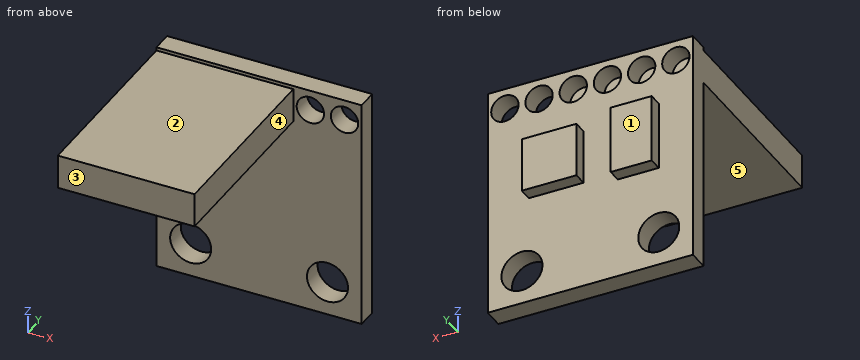
from build123d import *

# Parameters (mm, degrees)
ESQUISSE1_W        = 15
ESQUISSE1_H        = 17
ESQUISSE1_R        = 1.5
ESQUISSE1_R_2      = 1
BOSS_EXTRU_1_DEPTH = 1.5
ESQUISSE2_W        = 3
ESQUISSE2_H        = 5
ESQUISSE2_W_2      = 4
ESQUISSE2_H_2      = 4
BOSS_EXTRU_2_DEPTH = 1
ESQUISSE3_W        = 10
ESQUISSE3_H        = 2.5
BOSS_EXTRU_3_DEPTH = 14


with BuildPart() as part:
    # Esquisse1 → Boss.-Extru.1 (new body)
    with BuildSketch(Plane(origin=(0, 0, 0), x_dir=(1, 0, 0), z_dir=(0, 1, 0))):
        Rectangle(ESQUISSE1_W, ESQUISSE1_H)
        with Locations((-5, 6)):
            Circle(ESQUISSE1_R, mode=Mode.SUBTRACT)
        with Locations((5, 6)):
            Circle(ESQUISSE1_R, mode=Mode.SUBTRACT)
        with Locations((-6.25, -7)):
            Circle(ESQUISSE1_R_2, mode=Mode.SUBTRACT)
        with Locations((-3.75, -7)):
            Circle(ESQUISSE1_R_2, mode=Mode.SUBTRACT)
        with Locations((-1.25, -7)):
            Circle(ESQUISSE1_R_2, mode=Mode.SUBTRACT)
        with Locations((1.25, -7)):
            Circle(ESQUISSE1_R_2, mode=Mode.SUBTRACT)
        with Locations((3.75, -7)):
            Circle(ESQUISSE1_R_2, mode=Mode.SUBTRACT)
        with Locations((6.25, -7)):
            Circle(ESQUISSE1_R_2, mode=Mode.SUBTRACT)
    extrude(amount=BOSS_EXTRU_1_DEPTH)

    # Esquisse2 → Boss.-Extru.2 (add)
    with BuildSketch(Plane(origin=(0, 1.5, 0), x_dir=(1, 0, 0), z_dir=(0, 1, 0))):
        with Locations((-3.5, -1.5)):
            Rectangle(ESQUISSE2_W, ESQUISSE2_H)
        with Locations((2.5, -1.5)):
            Rectangle(ESQUISSE2_W_2, ESQUISSE2_H_2)
    extrude(amount=BOSS_EXTRU_2_DEPTH)

    # Esquisse3 → Boss.-Extru.3 (add)
    with BuildSketch(Plane.XZ):
        with Locations((-2.5, 7)):
            Rectangle(ESQUISSE3_W, ESQUISSE3_H)
    extrude(amount=BOSS_EXTRU_3_DEPTH)


solid = part.part
For this review, take the finished solid that the model builds, in its own axes (mm). Face numbers are marked on the shaded views. A direction names the side the tool comes from. Round coordinates to 2 decimals unless told otherwise and drop trailing zeros. Loops run counter-clockwise (first coordinate to the right, second up) from the corner with the lowest first, then second, coordinate; pieces in that order, holes last. Notation, with made-up numbers: (-22, -25.75) - (-16, -25.75) arc R28 cw to (-16, -6.75) - close; hole circle Ø2 at (4.25, 5.25). An arc over 180 degrees is marked (long way). One line per item, written item: value. Start each with the question number.
Item 1: Take a section at C-C (x = 3.75). Give the boundary of the cut face in (y, z).
Item 2: Take a section at A-A (z = 7). State how many separate pieces and enclosed holes the cut face has, plus the area to 4 significant figures.
Item 3: Clearance check with flat-ended pins moving along their axes: pin 1 Ø1.5 at (x, z) = (-0.5, -3) entering from -Y; pin 2 Ø3 at (y, z) = (-3.5, 7) entering from +X; pin 3 Ø2.5 at (x, z) = (5, -6) entering from +Y; pin 4 Ø1 at (x, z) = (-4, 7) entering from +Y. State where each tip first meets the part, or that it passes through.
Item 4: Take a section at B-B (x = 1.25). Give the boundary of the cut face in (y, z).
Item 5: For the marked faces 1, 2, 3, 4 and 5, list the 3-axis set-ups (+Z, -Z, +X, -X, +Y, -Y) from which the entire face can be reached by the end or side of a thin tool; tool diameter is ignored.
Item 6: Take a section at D-D (z = 2). Give the boundary of the cut face in (x, y), plus the area to 3 significant figures.
Item 7: For L1, parallel to Z at x = -6.25, y = 1.25; L2, parallel to Z at x = 1.25, y = 0.35; L3, parallel to Y at x = 3.5, z = 5.5, list the stretches that pass through material, from the lowest coordinate up.
Answer below:
1. outline: (0, -8.5) - (1.5, -8.5) - (1.5, -6.83) - (0, -6.83) - close; (0, -5.17) - (1.5, -5.17) - (1.5, -0.5) - (2.5, -0.5) - (2.5, 3.5) - (1.5, 3.5) - (1.5, 6) - (0, 6) - close; (0, 8) - (1.5, 8) - (1.5, 8.5) - (0, 8.5) - close
2. separate pieces: 3
2. enclosed holes: 0
2. area: 144.5 mm2
3. pin 1: stops at y = 0
3. pin 2: stops at x = 2.5
3. pin 3: passes through
3. pin 4: stops at y = 0
4. outline: (-14, 5.75) - (0, 5.75) - (0, -8.5) - (1.5, -8.5) - (1.5, -0.5) - (2.5, -0.5) - (2.5, 3.5) - (1.5, 3.5) - (1.5, 6) - (0, 6) - (0, 8) - (1.5, 8) - (1.5, 8.5) - (0, 8.5) - (0, 8.25) - (-14, 8.25) - close
5. face 1: +Z, -Z, +X, -X, +Y
5. face 2: +Z, +X, -X, -Y
5. face 3: +Z, -Z, +X, -X, -Y
5. face 4: +Z, -Z, +X, -Y
5. face 5: -Z, +X, -X, -Y
6. outline: (-7.5, 0) - (7.5, 0) - (7.5, 1.5) - (4.5, 1.5) - (4.5, 2.5) - (0.5, 2.5) - (0.5, 1.5) - (-2, 1.5) - (-2, 2.5) - (-5, 2.5) - (-5, 1.5) - (-7.5, 1.5) - close
6. area: 29.5 mm2
7. L1: z = -8.5 to -6.83, -5.17 to 6, 8 to 8.5
7. L2: z = -8.5 to 6, 8 to 8.5
7. L3: y = 0 to 1.5
